```python
from build123d import *

# Parameters (mm, degrees)
CROQUIS1_R              = 1.949957096
CROQUIS1_W              = 3.899914193
CROQUIS1_H              = 20
CROQUIS1_W_2            = 3.931890122
SALIENTE_EXTRUIR1_DEPTH = 4
CROQUIS3_W              = 4
CROQUIS3_H              = 20
CORTAR_EXTRUIR2_DEPTH   = 18


with BuildPart() as part:
    # Croquis1 → Saliente-Extruir1 (new body)
    with BuildSketch(Plane.XY):
        Polygon((1.526053109, 36.234397526), (1.526053109, 45.984183007), (5.425967302, 45.984183007), (5.425967302, 70.846135986), (20.538134799, 70.846135986), (20.538134799, 74.746050179), (40.037705762, 74.746050179), (40.037705762, 70.846135986), (69.287062208, 70.846135986), (69.287062208, 74.746050179), (88.786633171, 74.746050179), (88.786633171, 70.846135986), (103.898800668, 70.846135986), (103.898800668, 45.984183007), (107.798714861, 45.984183007), (107.798714861, 36.234397526), (107.798714861, 26.484612044), (103.898800668, 26.484612044), (103.898800668, 2.110148339), (5.425967302, 2.110148339), (5.425967302, 26.484612044), (1.526053109, 26.484612044), align=None)
        with Locations((43.902907702, 28.411154562)):
            Circle(CROQUIS1_R, mode=Mode.SUBTRACT)
        with Locations((72.35718349, 35.603908164)):
            Rectangle(CROQUIS1_W, CROQUIS1_H, mode=Mode.SUBTRACT)
        with Locations((95.740680681, 35.603908164)):
            Rectangle(CROQUIS1_W_2, CROQUIS1_H, mode=Mode.SUBTRACT)
    extrude(amount=SALIENTE_EXTRUIR1_DEPTH)

    # Croquis3 → Cortar-Extruir2 (cut)
    with BuildSketch(Plane.XY.offset(4)):
        with Locations((64.674115468, 37.164302326)):
            Rectangle(CROQUIS3_W, CROQUIS3_H)
        with Locations((25.674115468, 37.164302326)):
            Rectangle(CROQUIS3_W, CROQUIS3_H)
    extrude(amount=-CORTAR_EXTRUIR2_DEPTH, mode=Mode.SUBTRACT)


solid = part.part
```
CAD build for the part. Positions are in the model's coordinates, mm. A direction names the side the tool comes from. Round coordinates to 2 decimals unless told otherwise and drop trailing zeros. Write each loop counter-clockwise with the first axis right and the second up, starting at its lowest first coordinate (ties: lowest second). Pieces come first, ordered by that corner, then holes.
Item 1: Band-saw the part on C-C on y = 9.5. Write the cut outline in (x, z).
Filled in:
outline: (5.43, 0) - (103.9, 0) - (103.9, 4) - (5.43, 4) - close
Item 2: Band-saw the part on D-D on z = 2.6. Give the number of separate pieces and of enclosed holes in the cut face, then the cut area to 3 significant figures.
Filled in:
separate pieces: 1
enclosed holes: 5
area: 6,740 mm2
Item 3: Tool access for faces 4 (the flat face through (106, 45.984, 2)), 5 (the flat face through (54, 70.846, 2)), 6 (the flat face through (106, 26.485, 2)), 7 (the flat face through (23.674, 37, 2)), 8 (the flat face through (5.426, 58, 2)): list every direction of +Z, -Z, +X, -X, +Y, -Y with a clear straight run to the whole face (end or side of a thin tool).
Filled in:
face 4: +Z, -Z, +X, +Y
face 5: +Z, -Z, +Y
face 6: +Z, -Z, +X, -Y
face 7: +Z, -Z
face 8: +Z, -Z, -X, +Y
Item 4: Band-saw the part on B-B on x = 65.5. Write the cut outline in (y, z), then the cut area to 3 significant figures.
Filled in:
outline: (2.11, 0) - (27.16, 0) - (27.16, 4) - (2.11, 4) - close; (47.16, 0) - (70.85, 0) - (70.85, 4) - (47.16, 4) - close
area: 195 mm2
Item 5: Drop flat-ended pins along their axis: pin 1 Ø1.5 at (y, z) = (11.5, 1) entering from -X; pin 2 Ø2 at (x, z) = (16.5, 1.5) entering from +Y; pin 3 Ø1 at (y, z) = (18.5, 1.5) entering from +X; pin 4 Ø12 at (x, y) = (96, 27.5) entering from -Z. Give the stop position or say it passes through.
Filled in:
pin 1: stops at x = 5.43
pin 2: stops at y = 70.85
pin 3: stops at x = 103.9
pin 4: stops at z = 0
Item 6: Mould opens along X. For faces 1 (the flat face through (4, 26.485, 2)), 2 (the flat face through (72, 25.604, 2)), 3 (the flat face through (107.799, 36, 2)) say: released by +X, released by -X, zero draft, split by the parting line, or undercut.
Filled in:
face 1: zero draft
face 2: undercut
face 3: released by +X
Item 7: Drill centre lines: L1, parallel to X at y = 41, z = 1.6; L2, parallel to X at y = 71.5, z = 1.8; L3, parallel to Y at x = 24.5, z = 1.4. Where is each one in solid material? Low to high.
Filled in:
L1: x = 1.53 to 23.67, 27.67 to 62.67, 66.67 to 70.41, 74.31 to 93.77, 97.71 to 107.8
L2: x = 20.54 to 40.04, 69.29 to 88.79
L3: y = 2.11 to 27.16, 47.16 to 74.75
Item 8: Band-saw the part on A-A on y = 39.5. Write the cut outline in (x, z), then the cut area to 3 significant figures.
Filled in:
outline: (1.53, 0) - (23.67, 0) - (23.67, 4) - (1.53, 4) - close; (27.67, 0) - (62.67, 0) - (62.67, 4) - (27.67, 4) - close; (66.67, 0) - (70.41, 0) - (70.41, 4) - (66.67, 4) - close; (74.31, 0) - (93.77, 0) - (93.77, 4) - (74.31, 4) - close; (97.71, 0) - (107.8, 0) - (107.8, 4) - (97.71, 4) - close
area: 362 mm2
